```python
from build123d import *

# Parameters (mm, degrees)
BASE_FLANGE2_DEPTH = 1.5875
EDGE_FLANGE2_DEPTH = 43.999999884
FILLET2_R          = 1.27
SKETCH21_R         = 2
CUT_EXTRUDE1_DEPTH = 37.554305105


# Sheet-metal steps are written as plain solids
with BuildPart() as part:
    # Sketch12 → Base-Flange2 (new body)
    with BuildSketch(Plane(origin=(0, 0, 0), x_dir=(1, 0, 0), z_dir=(0, 1, 0))):
        with BuildLine():
            Line((-21.999999942, -33), (0, -33))
            Line((0, -33), (21.999999942, -33))
            Line((21.999999942, -33), (10.16, -7.62))
            ThreePointArc((10.16, -7.62), (0, -12.7), (-10.16, -7.62))
            Line((-10.16, -7.62), (-21.999999942, -33))
        make_face()
    extrude(amount=-BASE_FLANGE2_DEPTH)

    # Edge-Flange2 section (across the edge) → Edge-Flange2 (add)
    with BuildSketch(Plane(origin=(-21.999999942, 0, 34.27), x_dir=(0, 0, -1), z_dir=(1, 0, 0))):
        with BuildLine():
            Line((-1.5875, 1), (-1.5875, 14))
            Line((-1.5875, 14), (0, 14))
            Line((0, 14), (0, 1))
            ThreePointArc((0, 1), (0.292893219, 0.292893219), (1, 0))
            Line((1, 0), (1.27, 0))
            Line((1.27, 0), (1.27, -1.5875))
            Line((1.27, -1.5875), (1, -1.5875))
            ThreePointArc((1, -1.5875), (-0.829638796, -0.829638796), (-1.5875, 1))
        make_face()
    extrude(amount=EDGE_FLANGE2_DEPTH)

    # Fillet2
    fillet2_edges = [part.edges().sort_by_distance(p)[0] for p in [
        (-21.999999942, 14, 35.06375),
        (21.999999942, 14, 35.06375),
        (-10.16, -0.79375, 7.62),
        (10.16, -0.79375, 7.62),
    ]]
    fillet(fillet2_edges, radius=FILLET2_R)

    # Sketch21 → Cut-Extrude1 (cut, through all)
    with BuildSketch(Plane(origin=(0, 0, 34.27), x_dir=(-1, 0, 0), z_dir=(0, 0, -1))):
        with Locations((-17.5, 6.865)):
            Circle(SKETCH21_R)
        with Locations((17.5, 6.865)):
            Circle(SKETCH21_R)
    extrude(amount=-CUT_EXTRUDE1_DEPTH, mode=Mode.SUBTRACT)


solid = part.part
```
The model under review builds one solid part; all positions refer to its coordinate system, in mm. A direction names the side the tool comes from. Give positions to 0.01 mm unless a question says otherwise; leave off trailing zeros. Write each loop counter-clockwise with the first axis right and the second up, starting at its lowest first coordinate (ties: lowest second). Pieces come first, ordered by that corner, then holes. Notation, with made-up numbers: (-12, 41.25) - (-3, 41.25) arc R21 cw to (-3, 72.25) - close; hole circle Ø8 at (40.25, 32.5). An arc over 180 degrees is marked (long way). Answer in a Markdown table with one row per item. Add a question column.
1. We need section D-D on y = 1.5. Write out the cut boundary in (x, z), then the cut area to 4 significant figures.
2. Tool access review of faces 4 (the flat face through (0, 8, 34.27)), 5 (the cylindrical face through (-0.31, -0.85, 35.08)): name each direction out of +Z, -Z, +X, -X, +Y, -Y from which nothing blocks a thin tool from reaching the whole face with its end or side.
3. Insertion check: P1, Ø2, axis at x = -12.5, z = 29, coming from the +Y side; P2, Ø6.5, axis at x = 11, y = 10.5, coming from the -Z side; P3, Ø8, axis at x = 0, y = 3.5, coming from the -Z side; P4, Ø3.5, axis at x = -17.5, y = 6.865, coming from the +Z side. Each pin has a flat end and moves straight along its axis. Give the tip position at first contact, or say it passes through.
4. We need section B-B on y = 8. Write out the cut boundary in (x, z).
5. We need section A-A on x = -17.5. Write out the cut boundary in (y, z) (1 decimal).
6. Wall thickness on line 1 along Y through (x, z) = (8.5, 23.25); line 2 along Y through (x, z) = (17.5, 35.5) (3 decimals); line 3 along Z through (x, y) = (13, 10.75): over which ranges is each line inside the solid? List them lowest first. Write a range as [from, to].
7. Draft analysis for pull direction Y (two halves, no side actions). For faces 1 (the cylindrical face through (19.09, 5.65, 35.05)), 2 (the cylindrical face through (-21.618, 13.638, 35.053)), 3 (the cylindrical face through (10.073, -0.805, 8.676)), state which applies: +Y half, -Y half, draft (parallel to the pull), parting line (faces both ways), or undercut.
8. We need section C-C on x = 3. Write out the cut boundary in (y, z) (1 decimal), then the cut area to 3 significant figures.
Ans:
| question | item | result |
|---|---|---|
| 1 | outline | (-22, 34.27) - (22, 34.27) - (22, 35.86) - (-22, 35.86) - close |
| 1 | area | 69.85 mm^2 |
| 2 | face 4 | -Z, +X, -X, +Y |
| 2 | face 5 | +Z, +X, -X, -Y |
| 3 | P1 | stops at y = 0 |
| 3 | P2 | stops at z = 34.27 |
| 3 | P3 | stops at z = 12.55 |
| 3 | P4 | passes through |
| 4 | outline | (-22, 34.27) - (-19.15, 34.27) - (-19.15, 35.86) - (-22, 35.86) - close; (-15.85, 34.27) - (15.85, 34.27) - (15.85, 35.86) - (-15.85, 35.86) - close; (19.15, 34.27) - (22, 34.27) - (22, 35.86) - (19.15, 35.86) - close |
| 5 | outline | (-1.6, 23.4) - (0, 23.4) - (0, 33.3) arc R1 cw to (1, 34.3) - (4.9, 34.3) - (4.9, 35.9) - (1, 35.9) arc R2.6 ccw to (-1.6, 33.3) - close; (8.9, 34.3) - (14, 34.3) - (14, 35.9) - (8.9, 35.9) - close |
| 6 | line 1 | y = [-1.59, 0] |
| 6 | line 2 | y = [-0.312, 4.865], [8.865, 14] |
| 6 | line 3 | z = [34.27, 35.86] |
| 7 | face 1 | undercut |
| 7 | face 2 | +Y half |
| 7 | face 3 | draft |
| 8 | outline | (-1.6, 12.3) - (0, 12.3) - (0, 33.3) arc R1 cw to (1, 34.3) - (14, 34.3) - (14, 35.9) - (1, 35.9) arc R2.6 ccw to (-1.6, 33.3) - close |
| 8 | area | 58.3 mm^2 |
